Input: part model. Units: mm. Frame: model coordinates. Face numbers are marked on the shaded views. A direction names the side the tool comes from. Give positions to 0.01 mm unless a question says otherwise; leave off trailing zeros. Loops run counter-clockwise (first coordinate to the right, second up) from the corner with the lowest first, then second, coordinate; pieces in that order, holes last. Notation, with made-up numbers: M -35.75,-18.5 L 20.25,-18.5 A10 cw 20.25,-8.5 Z; hole C 33.25,6 d10. An arc over 180 degrees is marked long. Answer as a JSON object with one key per item and string values. Group by question number.
1) Section query A-A on x = 0. Return loops of the section in (y, z) (3 decimals).
2) First-contact query: P1, Ø5.5, axis at x = -11, z = -98.5, coming from the +Y side; P2, Ø6.5, axis at y = 7.5, z = 107, coming from the +X side; P3, Ø4, axis at y = 18, z = 98.5, coming from the -X side. Flat tips, straight axial feed; report the tip coordinate or a pass-through.
3) Draft query along X for the marked faces 3, 4 and 5. Return one class per face: +X half, -X half, draft (parallel to the pull), parting line (faces both ways), or undercut.
4) Ray query, L1, parallel to X at y = 14.4, z = -98.5; L2, parallel to Z at x = 7.5, y = 17.5; L3, parallel to X at y = 4.25, z = 99.5 (3 decimals). Return the intervals inside material, ascending.
5) Access query for the marked faces 1 and 2. Directions: +Z, -Z, +X, -X, +Y, -Y. A direction counts if a zero-diameter tool reaches every point of the face in a straight line with its end or side. Return the directions, or none.
6) Section query B-B on y = 3.75. Count the separate pieces of the cut face and the enclosed holes in it, plus the area to 3 significant figures.
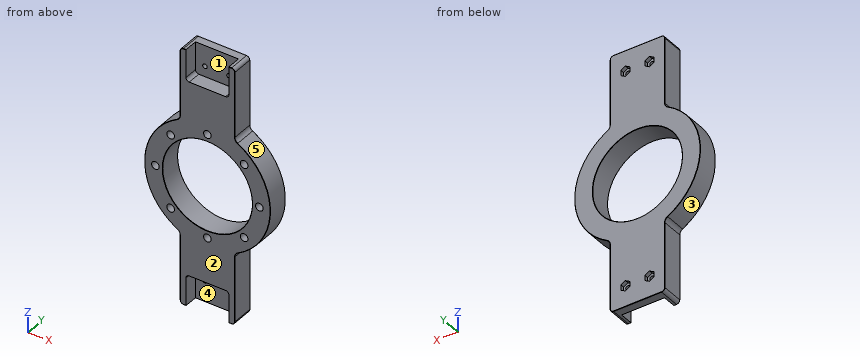
Autodesk Inventor part; units mm, degrees
ref_plane "YZ Plane" through (0, 0, 0) normal (1, 0, 0) x (0, 1, 0)
ref_plane "XZ Plane" through (0, 0, 0) normal (0, 1, 0) x (-1, 0, 0)
ref_plane "XY Plane" through (0, 0, 0) normal (0, 0, 1) x (1, 0, 0)
sketch "Sketch1" plane through (0, 0, 0) normal (0, 1, 0) x (-1, 0, 0)
  circle A0 centre (0, 0) radius 41
  line L0 (25, 117.5) -> (-25, 117.5)
  line L1 (-25, -117.5) -> (25, -117.5)
  arc A1 (-25, 51.7808) -> (-25, -51.7808) centre (0, 0) ccw
  arc A2 (25, -51.7808) -> (25, 51.7808) centre (0, 0) ccw
  line L2 (-25, 117.5) -> (-25, 51.7808)
  line L3 (-25, -51.7808) -> (-25, -117.5)
  line L4 (25, -117.5) -> (25, -51.7808)
  line L5 (25, 51.7808) -> (25, 117.5)
  dimension "d0" = 82
  dimension "d76" = 50
  dimension "d77" = 57.5
  dimension "d78" = 57.5
  dimension "d79" = 65.7192
  dimension "d80" = 65.7192
  dimension "d81" = 50
  dimension "d82" = 235
extrude "Extrusion1" add sketch "Sketch1" along normal blind 20
fillet "Fillet1" radius 5 4 edges at (-25, 10, 51.7808) (25, 10, 51.7808) (25, 10, -51.7808) (-25, 10, -51.7808)
fillet "Fillet2" radius 3 4 edges at (25, 10, 117.5) (-25, 10, 117.5) (25, 10, -117.5) (-25, 10, -117.5)
chamfer "Chamfer1" distance 0.25 angle 45 26 edges at (25, 20, 84.6646) (57.5, 20, 0) (25, 20, -84.6646) (24.1213, 20, -116.6213) (0, 20, -117.5) (-24.1213, 20, -116.6213) (-25, 20, -84.6646) (-57.5, 20, 0) (-25, 20, 84.6646) (-24.1213, 20, 116.6213) (0, 20, 117.5) (24.1213, 20, 116.6213) (25, 0, 84.6646) (57.5, 0, 0) (25, 0, -84.6646) (24.1213, 0, -116.6213) (0, 0, -117.5) (-24.1213, 0, -116.6213) (-25, 0, -84.6646) (-57.5, 0, 0) (-25, 0, 84.6646) (-24.1213, 0, 116.6213) (0, 0, 117.5) (24.1213, 0, 116.6213) (41, 20, 0) (41, 0, 0)
sketch "Sketch3" plane through (0, 0, 0) normal (0, -1, 0) x (1, 0, 0)
  line L0 (-22, -117.25) -> (-22, 117.25)
  line L1 (22, 117.25) -> (22, -117.25)
  line L2 (22, -117.25) -> (-22, 117.25) construction
  line L3 (-22, -117.25) -> (22, 117.25) construction
  line L4 (16.625, 89) -> (-16.625, 89)
  line L5 (-19.625, 92) -> (-19.625, 117.25)
  line L6 (19.625, 117.25) -> (19.625, 92)
  line L7 (19.625, 89) -> (17.4099, 92.7868) construction
  line L8 (-19.625, 89) -> (-17.1837, 91.5811) construction
  line L9 (-19.625, -117.25) -> (-19.625, -91.9916)
  line L10 (-16.6334, -88.9916) -> (16.6165, -88.8986)
  line L11 (19.6248, -91.8986) -> (19.6248, -117.25)
  line L12 (-17.2012, -91.6745) -> (-19.625, -89) construction
  line L13 (17.2501, -91.935) -> (19.6248, -88.8902) construction
  line L14 (22, 117.25) -> (19.625, 117.25)
  line L15 (-22, 117.5) -> (22, 117.5)
  line L16 (-19.625, 117.25) -> (-22, 117.25)
  arc A0 (-16.6334, -88.9916) -> (-19.625, -91.9916) centre (-16.625, -91.9916) ccw
  arc A1 (19.6248, -91.8986) -> (16.6165, -88.8986) centre (16.6248, -91.8986) ccw
  arc A2 (-19.625, 92) -> (-16.625, 89) centre (-16.625, 92) ccw
  arc A3 (16.625, 89) -> (19.625, 92) centre (16.625, 92) ccw
  line L17 (19.6248, -117.25) -> (19.6248, -121.1164)
  line L18 (19.6248, -121.1164) -> (-19.625, -121.1164)
  line L19 (-19.625, -121.1164) -> (-19.625, -117.25)
  line L20 (19.625, 117.25) -> (19.625, 123.825)
  line L21 (19.625, 123.825) -> (-19.625, 123.825)
  line L22 (-19.625, 123.825) -> (-19.625, 117.25)
  line L23 (19.625, 117.25) -> (19.6248, 117.25)
  line L24 (22, -117.25) -> (19.6248, -117.25)
  line L25 (-19.625, -117.25) -> (-22, -117.25)
  point P0 (0, 0)
  point P1 (-19.625, 117.5)
  point P2 (19.625, 117.5)
  dimension "d35" = 39.25
  dimension "d37" = 28.25
  dimension "d38" = 28.25
  dimension "d39" = 39.25
  dimension "d40" = 3
  dimension "d41" = 3
  dimension "d42" = 3
  dimension "d50" = 2.375
  dimension "d51" = 2.375
  dimension "d52" = 44
  dimension "d53" = 39.2499
  dimension "d55" = 2.3752
  dimension "d56" = 2.375
  dimension "d83" = 234.5
extrude "Extrusion4" cut sketch "Sketch3" against normal blind 12.575 contours L9 A0 L10 A1 L11 L17 L18 L19 | L22 L15 L20 L6 A3 L4 A2 L5 | L22 L21 L20 L15
sketch "Sketch4" plane through (0, 12.575, 0) normal (0, -1, 0) x (1, 0, 0)
  circle A0 centre (11, 98.5) radius 2.2451
  circle A1 centre (-11, 98.5) radius 2.3292
  circle A2 centre (10.9998, -98.5) radius 1.5784
  circle A3 centre (-11.0002, -98.5) radius 2.3162
  line L0 (19.6248, -117.5) -> (-19.625, -117.5)
  line L1 (-19.625, -117.5) -> (-19.625, -91.9916)
  line L2 (19.6248, -91.8986) -> (19.6248, -117.5)
  line L3 (-19.625, 117.5) -> (19.625, 117.5)
  line L4 (19.625, 117.25) -> (19.625, 92)
  point P0 (0, 0)
  point P1 (-19.625, -117.25)
  point P2 (19.6248, -117.25)
  dimension "d45" = 19
  dimension "d48" = 19
  dimension "d57" = 19
  dimension "d58" = 19
  dimension "d59" = 22
  dimension "d60" = 22
  dimension "d61" = 8.625
  dimension "d62" = 8.625
  dimension "d92" = 4.4901
hole "Hole2" at (11, 12.575, 98.5) at (-11, 12.575, 98.5) at (10.9998, 12.575, -98.5) at (-11.0002, 12.575, -98.5) direction (0, 1, 0) diameter 4.134 end through all
sketch "Sketch5" plane through (0, 20, 0) normal (0, 1, 0) x (1, 0, 0)
  circle A0 centre (-11, -98.5) radius 2.067
  line L0 (-11, -93.7369) -> (-6.875, -96.1184)
  line L1 (-6.875, -96.1184) -> (-6.875, -100.8816)
  line L2 (-6.875, -100.8816) -> (-11, -103.2631)
  line L3 (-11, -103.2631) -> (-15.125, -100.8816)
  line L4 (-15.125, -100.8816) -> (-15.125, -96.1184)
  line L5 (-15.125, -96.1184) -> (-11, -93.7369)
  circle A1 centre (11, -98.5) radius 2.067
  line L6 (11, -93.7369) -> (15.125, -96.1184)
  line L7 (15.125, -96.1184) -> (15.125, -100.8816)
  line L8 (15.125, -100.8816) -> (11, -103.2631)
  line L9 (11, -103.2631) -> (6.875, -100.8816)
  line L10 (6.875, -100.8816) -> (6.875, -96.1184)
  line L11 (6.875, -96.1184) -> (11, -93.7369)
  circle A2 centre (-11.0002, 98.5) radius 2.067
  line L12 (-11.0002, 93.7369) -> (-15.1252, 96.1184)
  line L13 (-15.1252, 96.1184) -> (-15.1252, 100.8816)
  line L14 (-15.1252, 100.8816) -> (-11.0002, 103.2631)
  line L15 (-11.0002, 103.2631) -> (-6.8752, 100.8816)
  line L16 (-6.8752, 100.8816) -> (-6.8752, 96.1184)
  line L17 (-6.8752, 96.1184) -> (-11.0002, 93.7369)
  circle A3 centre (10.9998, 98.5) radius 2.067
  line L18 (10.9998, 103.2631) -> (15.1248, 100.8816)
  line L19 (15.1248, 100.8816) -> (15.1248, 96.1184)
  line L20 (15.1248, 96.1184) -> (10.9998, 93.7369)
  line L21 (10.9998, 93.7369) -> (6.8748, 96.1184)
  line L22 (6.8748, 96.1184) -> (6.8748, 100.8816)
  line L23 (6.8748, 100.8816) -> (10.9998, 103.2631)
  point P0 (0, 0)
  point P1 (-13.0625, -102.0724)
  point P2 (-8.9377, 94.9276)
  dimension "d70" = 8.25
  dimension "d71" = 8.25
  dimension "d72" = 8.25
  dimension "d73" = 8.25
extrude "Extrusion5" cut sketch "Sketch5" against normal blind 3.45
sketch "Sketch6" plane through (0, 0, 0) normal (0, -1, 0) x (1, 0, 0)
  circle A0 centre (0, 0) radius 47.5
  circle A1 centre (0, -47.5) radius 3.5
  circle A2 centre (33.5876, -33.5876) radius 3.5
  circle A3 centre (47.5, 0) radius 3.5
  circle A4 centre (33.5876, 33.5876) radius 3.5
  circle A5 centre (0, 47.5) radius 3.5
  circle A6 centre (-33.5876, 33.5876) radius 3.5
  circle A7 centre (-47.5, 0) radius 3.5
  circle A8 centre (-33.5876, -33.5876) radius 3.5
  dimension "d84" = 95
  dimension "d85" = 7
  dimension "d88" = 360
extrude "Extrusion6" cut sketch "Sketch6" against normal blind 7 contours A0 A3 | A0 A3 | A4 A0 | A0 A4 | A2 A0 | A0 A2 | A5 A0 | A0 A5 | A1 A0 | A0 A1 | A6 A0 | A0 A6 | A8 A0 | A0 A8 | A7 A0 | A0 A7
properties part number "Head Thing"
Output:
{
 "1": {"outline": "M 0,-88.945 L 12.575,-88.945 L 12.575,-117.5 L 19.75,-117.5 L 20,-117.25 L 20,-41.25 L 19.75,-41 L 0.25,-41 L 0,-41.25 L 0,-44 L 7,-44 L 7,-51 L 0,-51 Z; M 0,41.25 L 0.25,41 L 19.75,41 L 20,41.25 L 20,117.25 L 19.75,117.5 L 12.575,117.5 L 12.575,89 L 0,89 L 0,51 L 7,51 L 7,44 L 0,44 Z"},
 "2": {"P1": "stops at y = 16.55", "P2": "stops at x = 25", "P3": "stops at x = -25"},
 "3": {"face 3": "-X half", "face 4": "undercut", "face 5": "+X half"},
 "4": {"L1": "x = -25 to -13.07, -8.93 to 8.93, 13.07 to 25", "L2": "z = -117.5 to -101.24, -95.76 to -40.31, 40.31 to 95.76, 101.24 to 117.5", "L3": "x = -25 to -19.625, 19.625 to 25"},
 "5": {"face 1": "+Z, -Y", "face 2": "+Z, -Z, +X, -X, -Y"},
 "6": {"separate pieces": "1", "enclosed holes": "9", "area": "8,750 mm^2"}
}
